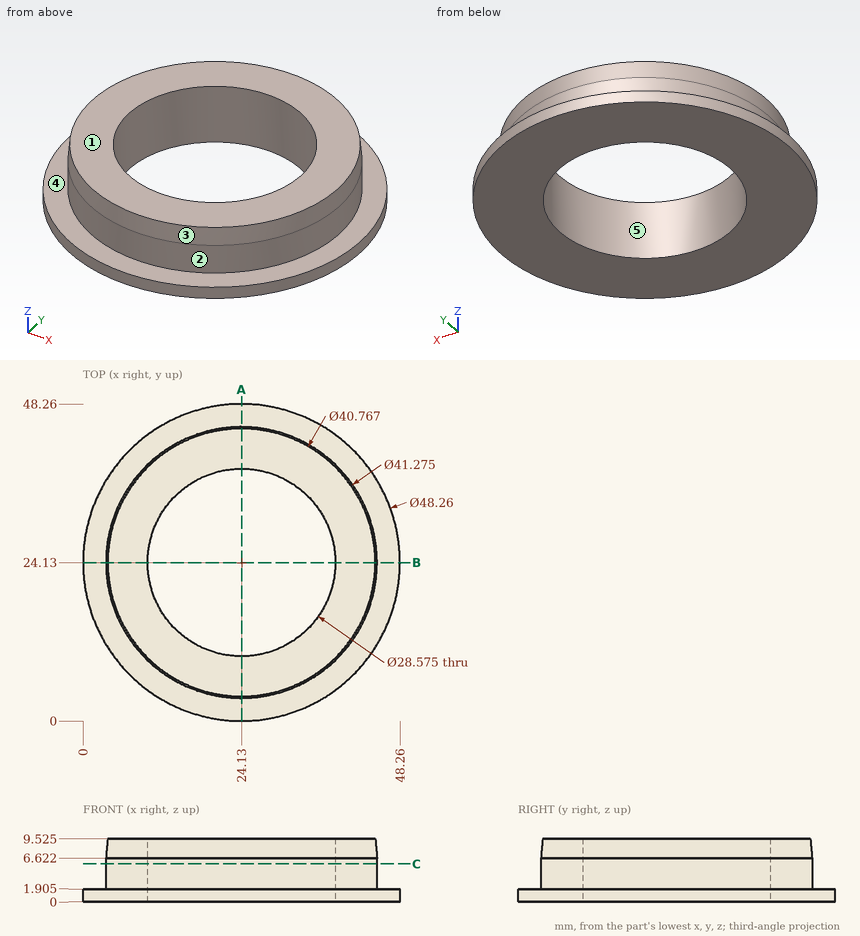
Geometry: see drawing. Coordinates: mm, zero at the bounding-box minimum. A direction names the side the tool comes from. Round coordinates to 2 decimals unless told otherwise and drop trailing zeros. Loops run counter-clockwise (first coordinate to the right, second up) from the corner with the lowest first, then second, coordinate; pieces in that order, holes last. Notation, with made-up numbers: (81.5, -28.75) -> (134.5, -28.75) arc R22 ccw to (134.5, 3.25) -> close; hole circle Ø1 at (46, -13.75). An arc over 180 degrees is marked (long way). One line per question, with ' | ' between items. Start each with the question number.
1. Section C-C on z = 5.75. Output: boundary loops of the cut face in (x, y) (1 decimal), and give its area (3 significant figures).
2. Mould query, pull axis Y, two halves, no side actions, for the marked faces 3, 4 and 5. Classes: pulls with the +Y half, pulls with the -Y half, needs draft (parallel to the pull), parting line crosses it, or undercut.
3. Contact query for flat-ended pins moving along their axis: pin 1 (10 mm diameter, centred on x = 6.5, y = 23, fed in from -Z); pin 2 (17 mm diameter, centred on x = 24.13, y = 24.13, fed in from -Z); pin 3 (5 mm diameter, centred on y = 43, z = 5.5, fed in from +X); pin 4 (1 mm diameter, centred on x = 11.5, z = 2, fed in from +Y). Output: stop coordinate, or through.
4. Set-up query: the marked faces 1 and 2. Return all of +Z, -Z, +X, -X, +Y, -Y with unobstructed straight access to the full face (end or side cutting, diameter ignored); none if empty.
5. Section A-A on x = 24.13. Output: boundary loops of the cut face in (y, z) (1 decimal).
6. Line query: line 1 along Y through (x, z) = (24.13, 2); line 2 along Z through (x, y) = (19.5, 46) (3 decimals); line 3 along Y through (x, z) = (24.13, 7.5). Output: solid intervals per line, ascending. Write a range as [from, to].
Returned:
1) outline: circle Ø41.3 at (24.1, 24.1); hole circle Ø28.6 at (24.1, 24.1) | area: 697 mm2
2) face 3: parting line crosses it | face 4: needs draft | face 5: undercut
3) pin 1: stops at z = 0 | pin 2: passes through | pin 3: stops at x = 36.7 | pin 4: stops at y = 44.98
4) face 1: +Z, +X, -X, +Y, -Y | face 2: +Z
5) outline: (0, 0) -> (9.8, 0) -> (9.8, 9.5) -> (3.7, 9.5) -> (3.5, 6.6) -> (3.5, 1.9) -> (0, 1.9) -> close; (38.4, 0) -> (48.3, 0) -> (48.3, 1.9) -> (44.8, 1.9) -> (44.8, 6.6) -> (44.5, 9.5) -> (38.4, 9.5) -> close
6) line 1: y = [3.49, 9.84], [38.42, 44.77] | line 2: z = [0, 1.905] | line 3: y = [3.57, 9.84], [38.42, 44.69]
